Check sheet for the drawn part. Datum: minimum x, y, z corner. Units: mm. A direction names the side the tool comes from. Give positions to 0.01 mm unless a question says otherwise; leave off trailing zeros. Write each loop counter-clockwise with the first axis right and the second up, starting at its lowest first coordinate (ties: lowest second). Pieces come first, ordered by that corner, then holes.
(1) Cross-section at D-D (z = 65.5). Record the boundary of the cut face in (x, y), and give its area (3 significant figures).
(2) Depth check by flat-ended pin: P1, Ø12, axis at x = 79, z = 10.5, coming from the -Y side; P2, Ø1, axis at y = 50, z = 18.5, coming from the +X side; P3, Ø8, axis at x = 46, z = 40, coming from the -Y side; P4, Ø1, axis at x = 43, y = 22, coming from the +Z side. Enter the tip coordinate at first touch or a pass-through.
(3) Cross-section at A-A (x = 53.1). Record the boundary of the cut face in (y, z).
(4) Thickness scan on line 1 along Z through (x, y) = (56.5, 10); line 2 along Z through (x, y) = (27.5, 8.5); line 3 along X through (y, z) = (90.5, 65). Record the ranges inside material, lowest first.
(5) Cross-section at C-C (z = 7). Record the boundary of the cut face in (x, y).
(6) Tool access check on the marked faces 1 and 2. Record the directions out of +Z, -Z, +X, -X, +Y, -Y that give a thin tool (end or side, any length) a straight path to the whole face; none if there is none.
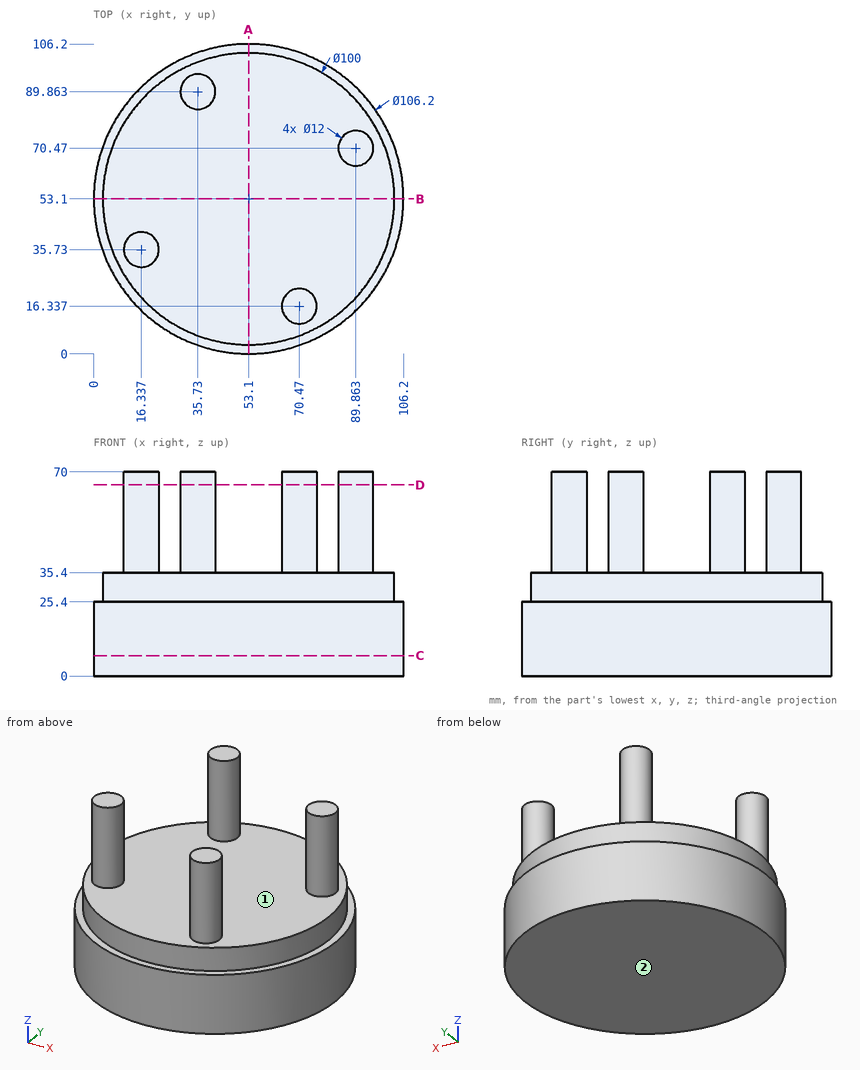
Reply:
1. outline: circle Ø12 at (16.34, 35.73); circle Ø12 at (35.73, 89.86); circle Ø12 at (70.47, 16.34); circle Ø12 at (89.86, 70.47)
1. area: 452 mm2
2. P1: stops at y = 3.87
2. P2: stops at x = 106.14
2. P3: passes through
2. P4: stops at z = 35.4
3. outline: (0, 0) - (106.2, 0) - (106.2, 25.4) - (103.1, 25.4) - (103.1, 35.4) - (3.1, 35.4) - (3.1, 25.4) - (0, 25.4) - close
4. line 1: z = 0 to 35.4
4. line 2: z = 0 to 25.4
4. line 3: x = 29.76 to 41.7
5. outline: circle Ø106.2 at (53.1, 53.1)
6. face 1: +Z
6. face 2: -Z, +X, -X, +Y, -Y
